Input: part model. Units: mm. Frame: model coordinates. Give positions to 0.01 mm unless a question says otherwise; leave off trailing zeros. Loops run counter-clockwise (first coordinate to the right, second up) from the corner with the lowest first, then second, coordinate; pieces in that order, holes last. Notation, with made-up numbers: (-22.75, 79) -> (32.25, 79) arc R21 cw to (32.25, 86) -> close; hole circle Ø9 at (32.5, -33.5). An arc over 180 degrees is marked (long way). Answer as a JSON object with one key per item and string values. Group by question number.
```python
from build123d import *

# Parameters (mm, degrees)
BOSS_EXTRUDE1_DEPTH = 15.6


with BuildPart() as part:
    # Sketch2 → Boss-Extrude1 (new body)
    with BuildSketch(Plane(origin=(0, 0, 0), x_dir=(0, 0, -1), z_dir=(1, 0, 0))):
        Polygon((0.2, 47.3), (0.1, 47.3), (0.1, 3.5), (0.2, 3.5), (0.2, 0), (0, 0), (0, 3.5), (0, 47.3), (0, 50.8), (0.2, 50.8), align=None)
    extrude(amount=-BOSS_EXTRUDE1_DEPTH)


solid = part.part
```
Q1. Section B-B on x = -9.5. Return the cut outline in (y, z).
Q2. Section C-C on y = 37. Return the cut outline in (x, z), then the cut area to 3 significant figures.
Q3. Pin query (flat end, axial travel): pin 1 Ø4.5 at (x, y) = (-5, 33.5) entering from -Z. Return the tip coordinate at first contact, or that it passes through.
Q4. Section A-A on z = -0.15. Return the cut outline in (x, y).
Q5. Ray query, probe 1 along Y at (x, z) = (-4.25, -0.15). Return the intervals inside material, ascending.
Numbers:
{
 "1": {"outline": "(0, -0.2) -> (3.5, -0.2) -> (3.5, -0.1) -> (47.3, -0.1) -> (47.3, -0.2) -> (50.8, -0.2) -> (50.8, 0) -> (0, 0) -> close"},
 "2": {"outline": "(-15.6, -0.1) -> (0, -0.1) -> (0, 0) -> (-15.6, 0) -> close", "area": "1.56 mm²"},
 "3": {"pin 1": "stops at z = -0.1"},
 "4": {"outline": "(-15.6, 0) -> (0, 0) -> (0, 3.5) -> (-15.6, 3.5) -> close; (-15.6, 47.3) -> (0, 47.3) -> (0, 50.8) -> (-15.6, 50.8) -> close"},
 "5": {"probe 1": "y = 0 to 3.5, 47.3 to 50.8"}
}
